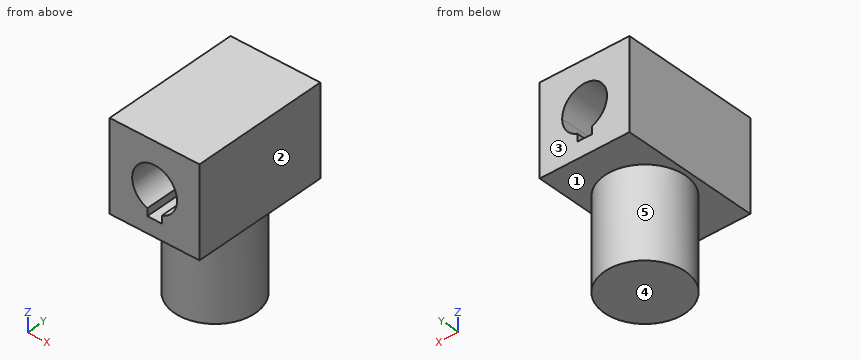
from build123d import *

# Parameters (mm, degrees)
SKETCH1_W           = 50
SKETCH1_H           = 50
BOSS_EXTRUDE1_DEPTH = 77
SKETCH2_R           = 22.5
BOSS_EXTRUDE2_DEPTH = 50


with BuildPart() as part:
    # Sketch1 → Boss-Extrude1 (new body)
    with BuildSketch(Plane(origin=(0, 0, 0), x_dir=(1, 0, 0), z_dir=(0, 1, 0))):
        Rectangle(SKETCH1_W, SKETCH1_H)
        with BuildLine():
            Line((4, 16), (4, 11.842719282))
            ThreePointArc((4, 11.842719282), (10.155048006, 7.288689869), (12.5, 0))
            ThreePointArc((12.5, 0), (-7.288689869, -10.155048006), (-4, 11.842719282))
            Line((-4, 11.842719282), (-4, 16))
            Line((-4, 16), (4, 16))
        make_face(mode=Mode.SUBTRACT)
    extrude(amount=BOSS_EXTRUDE1_DEPTH)

    # Sketch2 → Boss-Extrude2 (add)
    with BuildSketch(Plane(origin=(0, 0, -25), x_dir=(-1, 0, 0), z_dir=(0, 0, -1))):
        with Locations((0, 38.5)):
            Circle(SKETCH2_R)
    extrude(amount=BOSS_EXTRUDE2_DEPTH)


solid = part.part
Can you work these out from the model? Positions are in its coordinate system, mm. Face numbers are marked on the shaded views. A direction names the side the tool comes from. Coordinates: 2 decimals unless noted, no trailing zeros. Write each loop counter-clockwise with the first axis right and the second up, starting at its lowest first coordinate (ties: lowest second). Pieces come first, ordered by that corner, then holes. Notation, with made-up numbers: (1.5, 63) - (50.5, 63) arc R35 ccw to (50.5, 99) - close; hole circle Ø1 at (27.5, 46). An arc over 180 degrees is marked (long way). Return JSON: item names as keys, results as strings. Group by question number.
Item 1: If we section it at C-C (y = 38.5): Write out the boundary of the cut face in (x, z), then the cut area to 3 significant figures.
Item 2: If we section it at D-D (x = -17.5): Write out the boundary of the cut face in (y, z), then the cut area to 3 significant figures.
Item 3: We'd pull the mould along Y, two halves only. Please class the marked faces 3, 4 and 5: pulls with the +Y half, pulls with the -Y half, needs draft (parallel to the pull), parting line crosses it, or undercut.
Item 4: Which directions (+Z, -Z, +X, -X, +Y, -Y) give clear straight access to the entire face, cutting with the end or side of a thin tool? Please do the marked faces 1 and 2.
Item 5: I'm going to push flat-ended pins straight in: pin 1 Ø10 at (x, z) = (-1.5, 2.5) entering from +Y; pin 2 Ø2 at (x, z) = (-12, -37.5) entering from -Y. Where does each tip first touch, or does it pass through?
Item 6: If we section it at A-A (z = 10): Write out the boundary of the cut face in (x, y), then the cut area to 4 significant figures.
Item 7: Please list where these lines run through material, in increasing order: probe 1 along Z at (x, y) = (0, 46.5); probe 2 along Z at (x, y) = (15.5, 72.5); probe 3 along Z at (x, y) = (-10.5, 46.5).
Item 8: If we section it at B-B (x = 0): Write out the boundary of the cut face in (y, z), then the cut area to 3 significant figures.
Return value:
{
 "1": {"outline": "(-25, -25) - (-22.5, -25) - (-22.5, -75) - (22.5, -75) - (22.5, -25) - (25, -25) - (25, 25) - (-25, 25) - close; hole (-4, -16) - (4, -16) - (4, -11.84) arc R12.5 ccw (long way) to (-4, -11.84) - close", "area": "4,230 mm^2"},
 "2": {"outline": "(0, -25) - (24.36, -25) - (24.36, -75) - (52.64, -75) - (52.64, -25) - (77, -25) - (77, 25) - (0, 25) - close", "area": "5,260 mm^2"},
 "3": {"face 3": "pulls with the +Y half", "face 4": "needs draft", "face 5": "parting line crosses it"},
 "4": {"face 1": "-Z", "face 2": "+Z, -Z, +X, +Y, -Y"},
 "5": {"pin 1": "passes through", "pin 2": "stops at y = 18.87"},
 "6": {"outline": "(-25, 0) - (-7.5, 0) - (-7.5, 77) - (-25, 77) - close; (7.5, 0) - (25, 0) - (25, 77) - (7.5, 77) - close", "area": "2,695 mm^2"},
 "7": {"probe 1": "z = -75 to -16, 12.5 to 25", "probe 2": "z = -25 to 25", "probe 3": "z = -75 to -6.78, 6.78 to 25"},
 "8": {"outline": "(0, -25) - (16, -25) - (16, -75) - (61, -75) - (61, -25) - (77, -25) - (77, -16) - (0, -16) - close; (0, 12.5) - (77, 12.5) - (77, 25) - (0, 25) - close", "area": "3,910 mm^2"}
}
